```python
from build123d import *

# Parameters (mm, degrees)
F0_R     = 31.75
F1_DEPTH = 22.225
F2_T     = -2.54
F4_D     = 8.89
F4_DEPTH = 31.751
F5_D     = 8.89
F6_R     = 5.08


with BuildPart() as f1:
    # F0 (on Top) → F1 (new body, symmetric)
    with BuildSketch(Plane.XY):
        Circle(F0_R)
    extrude(amount=F1_DEPTH, both=True)

    # F2
    f2_openings = [f1.faces().sort_by_distance(p)[0] for p in [
        (0, 0, 22.225),
    ]]
    offset(amount=F2_T, openings=f2_openings)

    # F4 (through all, one way)
    with BuildSketch(Plane(origin=(0, 0, 0), x_dir=(1, 0, 0), z_dir=(0, 1, 0))):
        with Locations((0, -17.2211941394)):
            Circle(F4_D / 2)
    extrude(amount=-F4_DEPTH, mode=Mode.SUBTRACT)

    # F5 (through all)
    with Locations(Plane.XZ):
        with Locations((0, 17.2211941394)):
            Hole(F5_D / 2)

    # F6
    f6_edges = [f1.edges().sort_by_distance(p)[0] for p in [
        (-31.75, 0, -22.225),
    ]]
    fillet(f6_edges, radius=F6_R)


solid = f1.part
```
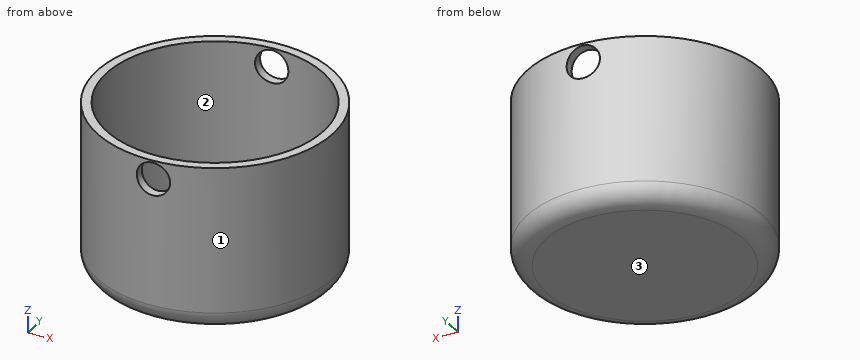
The listing builds one solid part. Answer for the finished solid, in the listing's coordinates (mm). Face numbers are marked on the shaded views. Coordinates: 2 decimals unless noted, no trailing zeros. Write each loop counter-clockwise with the first axis right and the second up, starting at its lowest first coordinate (ties: lowest second). Pieces come first, ordered by that corner, then holes. Notation, with made-up numbers: (-6, -23) - (19, -23) arc R34 ccw to (19, 9) - close; hole circle Ø5 at (-15.5, 82). An arc over 180 degrees is marked (long way). Return JSON: item names as keys, results as strings. Group by question number.
Q1. Flat-ended cylindrical pins translate along their axes: pin 1 Ø5.5 at (x, z) = (0, 17.22) entering from +Y; pin 2 Ø10 at (x, y) = (15, 8) entering from +Z (3 decimals); pin 3 Ø2 at (y, z) = (21.5, 17.5) entering from +X; pin 4 Ø2 at (x, z) = (10.5, 2.5) entering from -Y. Find the tip coordinate at first contact, or state that the pin passes through.
Q2. The part is cut by section B-B on z = 5. Write down the section's boundary in (x, y).
Q3. The part is cut by section A-A on x = 0. Write down the section's boundary in (y, z) (3 decimals).
Q4. For a pull along Y with two mould halves and no side action, classify the marked faces 1, 2 and 3 as +Y half, -Y half, draft (parallel to the pull), parting line (faces both ways), or undercut.
Q5. Find the intervals of material crossed by line 1 along Y through (x, z) = (0, -3); line 2 along Z through (x, y) = (-5, 6.5) (3 decimals); line 3 along Z through (x, y) = (0, 30.75) (3 decimals), in increasing order. Write a range as [from, to].
Q6. The part is cut by section C-C on y = 0. Write down the section's boundary in (x, z) (3 decimals).
Evaluation:
{
 "1": {"pin 1": "passes through", "pin 2": "stops at z = -19.685", "pin 3": "stops at x = 24.24", "pin 4": "stops at y = -30.3"},
 "2": {"outline": "circle Ø63.5 at (0, 0); hole circle Ø58.42 at (0, 0)"},
 "3": {"outline": "(-31.75, -17.145) arc R5.08 ccw to (-26.67, -22.225) - (26.67, -22.225) arc R5.08 ccw to (31.75, -17.145) - (31.75, 12.776) - (29.21, 12.776) - (29.21, -19.685) - (-29.21, -19.685) - (-29.21, 12.776) - (-31.75, 12.776) - close; (-31.75, 21.666) - (-29.21, 21.666) - (-29.21, 22.225) - (-31.75, 22.225) - close; (29.21, 21.666) - (31.75, 21.666) - (31.75, 22.225) - (29.21, 22.225) - close"},
 "4": {"face 1": "parting line", "face 2": "undercut", "face 3": "draft"},
 "5": {"line 1": "y = [-31.75, -29.21], [29.21, 31.75]", "line 2": "z = [-22.225, -19.685]", "line 3": "z = [-20.172, 12.776], [21.666, 22.225]"},
 "6": {"outline": "(-31.75, -17.145) arc R5.08 ccw to (-26.67, -22.225) - (26.67, -22.225) arc R5.08 ccw to (31.75, -17.145) - (31.75, 22.225) - (29.21, 22.225) - (29.21, -19.685) - (-29.21, -19.685) - (-29.21, 22.225) - (-31.75, 22.225) - close"}
}
